Could you check a few things on this model? Use its own coordinates, in mm. A direction names the side the tool comes from. Round coordinates to 2 decimals unless told otherwise and drop trailing zeros. Write each loop counter-clockwise with the first axis right and the second up, starting at its lowest first coordinate (ties: lowest second). Pieces come first, ordered by that corner, then holes. Notation, with made-up numbers: (40.25, -23) -> (88.25, -23) arc R25 ccw to (88.25, 3) -> close; hole circle Ø10 at (52.5, 80). An arc over 180 degrees is marked (long way). Answer in a Markdown table with one row per item.
from build123d import *

# Parameters (mm, degrees)
PAH1_SIZE                   = 2
KES_EKSTR_ZYON1_START       = 15
KES_EKSTR_ZYON1_DEPTH       = 10
KES_EKSTR_ZYON2_START       = 9
KES_EKSTR_ZYON2_DEPTH       = 10
M8X1_0_DI_LI_DELIK1_D       = 7
M8X1_0_DI_LI_DELIK1_DEPTH   = 28
M8X1_0_DI_LI_DELIK1_TIP     = 2.103012167
M10X1_25_DI_LI_DELIK1_D     = 8.8
M10X1_25_DI_LI_DELIK1_DEPTH = 28.75
M10X1_25_DI_LI_DELIK1_TIP   = 2.643786724


with BuildPart() as part:
    # Çizim1 → Döndür1 (revolve)
    with BuildSketch(Plane(origin=(0, 0, 0), x_dir=(1, 0, 0), z_dir=(0, 0, -1)), mode=Mode.PRIVATE) as d_nd_r1_sk:
        Polygon((0, 0), (225, 0), (225, 12.5), (163, 12.5), (163, 14.5), (145, 14.5), (145, 15), (127, 15), (127, 19), (105, 19), (105, 25), (100, 25), (100, 20), (42, 20), (42, 16), (17, 16), (17, 15), (0, 15), align=None)
    revolve(d_nd_r1_sk.sketch.rotate(Axis((0, 0, 0), (1, 0, 0)), 270), axis=Axis((0, 0, 0), (1, 0, 0)))

    # Pah1
    pah1_edges = [part.edges().sort_by_distance(p)[0] for p in [
        (225, 0, -12.5),
        (127, 0, -19),
        (42, 0, -20),
        (0, 0, -15),
    ]]
    chamfer(pah1_edges, length=PAH1_SIZE)

    # Çizim2 → Kes-Ekstrüzyon1 (cut)
    with BuildSketch(Plane(origin=(0, 0, 0), x_dir=(1, 0, 0), z_dir=(0, 1, 0)).offset(KES_EKSTR_ZYON1_START)):
        with BuildLine():
            Line((55, 6), (90, 6))
            ThreePointArc((90, 6), (96, 0), (90, -6))
            Line((90, -6), (55, -6))
            ThreePointArc((55, -6), (49, 0), (55, 6))
        make_face()
    extrude(amount=KES_EKSTR_ZYON1_DEPTH, mode=Mode.SUBTRACT)

    # Çizim3 → Kes-Ekstrüzyon2 (cut)
    with BuildSketch(Plane(origin=(0, 0, 0), x_dir=(1, 0, 0), z_dir=(0, 1, 0)).offset(KES_EKSTR_ZYON2_START)):
        with BuildLine():
            Line((173, 4), (210, 4))
            ThreePointArc((210, 4), (214, 0), (210, -4))
            Line((210, -4), (173, -4))
            ThreePointArc((173, -4), (169, 0), (173, 4))
        make_face()
    extrude(amount=KES_EKSTR_ZYON2_DEPTH, mode=Mode.SUBTRACT)

    # M8x1.0 Dişli Delik1
    with Locations(Plane(origin=(225, 0, 0), x_dir=(0, 0, -1), z_dir=(1, 0, 0))):
        with Locations((0, 0)):
            Hole(M8X1_0_DI_LI_DELIK1_D / 2, depth=M8X1_0_DI_LI_DELIK1_DEPTH)
            with Locations((0, 0, -(M8X1_0_DI_LI_DELIK1_DEPTH + M8X1_0_DI_LI_DELIK1_TIP / 2))):  # 118° drill point
                Cone(0, M8X1_0_DI_LI_DELIK1_D / 2, M8X1_0_DI_LI_DELIK1_TIP, mode=Mode.SUBTRACT)

    # M10x1.25 Dişli Delik1
    with Locations(Plane.ZY):
        with Locations((0, 0)):
            Hole(M10X1_25_DI_LI_DELIK1_D / 2, depth=M10X1_25_DI_LI_DELIK1_DEPTH)
            with Locations((0, 0, -(M10X1_25_DI_LI_DELIK1_DEPTH + M10X1_25_DI_LI_DELIK1_TIP / 2))):  # 118° drill point
                Cone(0, M10X1_25_DI_LI_DELIK1_D / 2, M10X1_25_DI_LI_DELIK1_TIP, mode=Mode.SUBTRACT)


solid = part.part
1) Imagine slicing it at C-C, the plane x = 92. Please give me the cut outline in (y, z).
Findings:
| item | result |
|---|---|
| outline | (15, -5.66) -> (15, 5.66) -> (19.18, 5.66) arc R20 ccw (long way) to (19.18, -5.66) -> close |
2) For pin 1 (2.5 mm diameter, centred on x = 194.5, z = -1, fed in from +Y); pin 2 (0.9 mm diameter, centred on x = 192, y = 11, fed in from -Z); pin 3 (1.5 mm diameter, centred on y = -3.5, z = -18, fed in from -X), each with a flat end and sliding along its axis, tell me the tip position at first contact or that it passes through.
Findings:
| item | result |
|---|---|
| pin 1 | stops at y = 9 |
| pin 2 | stops at z = -6.7 |
| pin 3 | stops at x = 42 |
3) For faces 4 (the face through (127, 14, -6)), 5 (the face through (14.576, 1.322, -4.197)), 6 (the face through (73, 17, 6)), which set-ups out of +Z, -Z, +X, -X, +Y, -Y let a thin tool reach every point of the face, with its end or its side?
Findings:
| item | result |
|---|---|
| face 4 | +X |
| face 5 | -X |
| face 6 | +Y |
4) Thinking about a two-plate mould opening in X: for faces 1 (the face through (224.875, -3.191, 10.134)), 2 (the face through (73, 15, 0)), 3 (the face through (135.874, -0.66, -14.985)), which applies, +X half, -X half, draft (parallel to the pull), parting line (faces both ways), or undercut?
Findings:
| item | result |
|---|---|
| face 1 | +X half |
| face 2 | undercut |
| face 3 | draft |
5) Imagine slicing it at B-B, the plane x = 155.5. Please give me the cut outline in (y, z).
Findings:
| item | result |
|---|---|
| outline | circle Ø29 at (0, 0) |
6) Please list where these lines run through material, in increasing order: line 1 (Y direction, x = 211, z = 0); line 2 (Y direction, x = 20, z = 0); line 3 (X direction, y = -15, z = -18).
Findings:
| item | result |
|---|---|
| line 1 | y = -12.5 to -3.5, 3.5 to 9 |
| line 2 | y = -16 to -4.4, 4.4 to 16 |
| line 3 | x = 100 to 105 |
7) Imagine slicing it at A-A, the plane x = 15. Please give me the cut outline in (y, z).
Findings:
| item | result |
|---|---|
| outline | circle Ø30 at (0, 0); hole circle Ø8.8 at (0, 0) |
